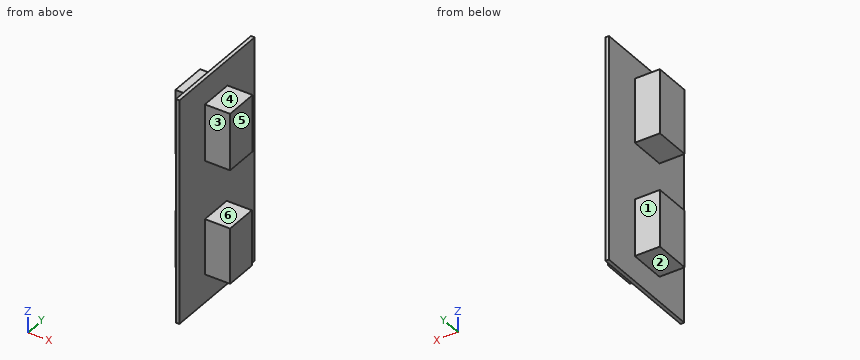
from build123d import *

# Parameters (mm, degrees)
CROQUIS1_W              = 500
CROQUIS1_H              = 250
SALIENTE_EXTRUIR1_DEPTH = 8
CROQUIS2_W              = 126.86716197
CROQUIS2_H              = 82.080673108
CROQUIS2_W_2            = 143.345907008
SALIENTE_EXTRUIR2_DEPTH = 56
CROQUIS4_W              = 126.86716197
CROQUIS4_H              = 82.080673108
SALIENTE_EXTRUIR4_DEPTH = 56
CROQUIS6_W              = 126.300102785
CROQUIS6_H              = 74.898758159
SALIENTE_EXTRUIR5_DEPTH = 56
CROQUIS7_W              = 123.680930687
CROQUIS7_H              = 72.443779117
SALIENTE_EXTRUIR6_DEPTH = 56


with BuildPart() as part:
    # Croquis1 → Saliente-Extruir1 (new body)
    with BuildSketch(Plane(origin=(0, 0, 0), x_dir=(0, 0, -1), z_dir=(1, 0, 0))):
        with Locations((-250, 125)):
            Rectangle(CROQUIS1_W, CROQUIS1_H)
    extrude(amount=SALIENTE_EXTRUIR1_DEPTH)

    # Croquis2 → Saliente-Extruir2 (add)
    with BuildSketch(Plane.ZY):
        with Locations((119.573923975, 123.338686018)):
            Rectangle(CROQUIS2_W, CROQUIS2_H)
        with Locations((381.283910617, 123.338686018)):
            Rectangle(CROQUIS2_W_2, CROQUIS2_H)
    extrude(amount=SALIENTE_EXTRUIR2_DEPTH)

    # Croquis4 → Saliente-Extruir4 (add)
    with BuildSketch(Plane.ZY):
        with Locations((119.573923975, 123.338686018)):
            Rectangle(CROQUIS4_W, CROQUIS4_H)
    extrude(amount=SALIENTE_EXTRUIR4_DEPTH)

    # Croquis6 → Saliente-Extruir5 (add)
    with BuildSketch(Plane(origin=(8, 0, 0), x_dir=(0, 0, -1), z_dir=(1, 0, 0))):
        with Locations((-380.044849003, 122.441200165)):
            Rectangle(CROQUIS6_W, CROQUIS6_H)
    extrude(amount=SALIENTE_EXTRUIR5_DEPTH)

    # Croquis7 → Saliente-Extruir6 (add)
    with BuildSketch(Plane(origin=(8, 0, 0), x_dir=(0, 0, -1), z_dir=(1, 0, 0))):
        with Locations((-124.804336035, 121.213710644)):
            Rectangle(CROQUIS7_W, CROQUIS7_H)
    extrude(amount=SALIENTE_EXTRUIR6_DEPTH)


solid = part.part
Part model, mm, in its own coordinate system. Face numbers are marked on the shaded views. A direction names the side the tool comes from. Coordinates: 2 decimals unless noted, no trailing zeros. Order: outer loops, then holes, each group sorted by start corner. A loop starts at its lowest first (then second) coordinate and runs counter-clockwise, first axis right, second up. Notation, with made-up numbers: M -24.5,-6.5 L -20.5,-6.5 A4 cw -20.5,0.5 Z; hole C -0.75,3 d9. An arc over 180 degrees is marked long. Use a Markdown table: item, result.
(1) Cut at C-C on z = 114. Write the cut outline in (x, y), then the cut area to 3 significant figures.
A:
| item | result |
|---|---|
| outline | M -56,82.3 L 0,82.3 L 0,0 L 8,0 L 8,84.99 L 64,84.99 L 64,157.44 L 8,157.44 L 8,250 L 0,250 L 0,164.38 L -56,164.38 Z |
| area | 10,700 mm^2 |
(2) Probe L1, parallel to Z at x = 49.5, y = 153.5; L2, parallel to X at y = 207.5, z = 255; L3, parallel to Y at x = 37, z = 415. List the from-to ranges inside material, lowest first.
A:
| item | result |
|---|---|
| L1 | z = 62.96 to 186.64, 316.89 to 443.19 |
| L2 | x = 0 to 8 |
| L3 | y = 84.99 to 159.89 |
(3) Cut at A-A on x = -33.5. Write the cut outline in (y, z).
A:
| item | result |
|---|---|
| outline | M 82.3,56.14 L 164.38,56.14 L 164.38,183.01 L 82.3,183.01 Z; M 82.3,309.61 L 164.38,309.61 L 164.38,452.96 L 82.3,452.96 Z |
(4) Flat gauge pins, fed straight in: pin 1 (17 mm diameter, centred on x = 50, z = 124, fed in from -Y); pin 2 (10 mm diameter, centred on x = 36.5, z = 407.5, fed in from +Y); pin 3 (8 mm diameter, centred on y = 60.5, z = 129.5, fed in from -X). Where does each tip first touch, or does it go through?
A:
| item | result |
|---|---|
| pin 1 | stops at y = 84.99 |
| pin 2 | stops at y = 159.89 |
| pin 3 | stops at x = 0 |
(5) Cut at B-B on y = 109. Write the cut outline in (x, z), then the cut area to 3 significant figures.
A:
| item | result |
|---|---|
| outline | M -56,56.14 L 0,56.14 L 0,0 L 8,0 L 8,62.96 L 64,62.96 L 64,186.64 L 8,186.64 L 8,316.89 L 64,316.89 L 64,443.19 L 8,443.19 L 8,500 L 0,500 L 0,452.96 L -56,452.96 L -56,309.61 L 0,309.61 L 0,183.01 L -56,183.01 Z |
| area | 33,100 mm^2 |
(6) Tool access for the marked faces 1, 2 and 3: list every direction of +Z, -Z, +X, -X, +Y, -Y with a clear straight run to the whole face (end or side of a thin tool).
A:
| item | result |
|---|---|
| face 1 | +Z, -Z, -X, +Y |
| face 2 | -Z, -X, +Y, -Y |
| face 3 | +Z, -Z, +X, -Y |
(7) Cut at D-D on x = 20.5. Write the cut outline in (y, z), then the cut area to 3 significant figures.
A:
| item | result |
|---|---|
| outline | M 84.99,62.96 L 157.44,62.96 L 157.44,186.64 L 84.99,186.64 Z; M 84.99,316.89 L 159.89,316.89 L 159.89,443.19 L 84.99,443.19 Z |
| area | 18,400 mm^2 |
(8) Pull direction Z, two halves, no side cores. Call the marked faces 4, 5 and 6: released by +Z, released by -Z, zero draft, split by the parting line, or undercut.
A:
| item | result |
|---|---|
| face 4 | released by +Z |
| face 5 | zero draft |
| face 6 | undercut |
